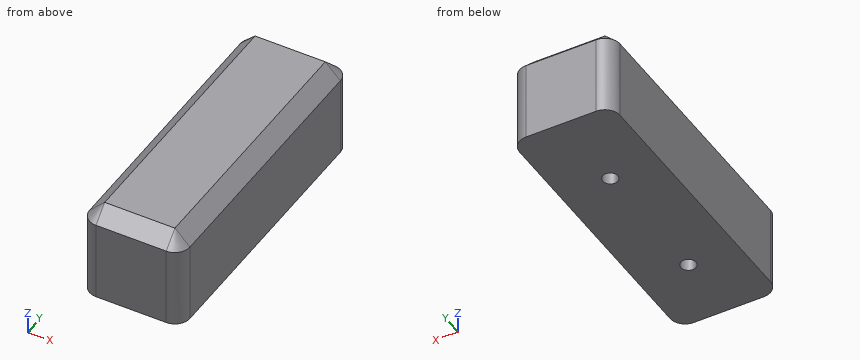
```python
from build123d import *

# Parameters (mm, degrees)
F0_W     = 20
F0_H     = 58
F1_DEPTH = 19
F2_R     = 1.5
F3_DEPTH = 17.000001
F4_R     = 3
F5_SIZE  = 3


with BuildPart() as f1:
    # F0 (on Top) → F1 (new body)
    with BuildSketch(Plane.XY):
        Rectangle(F0_W, F0_H)
    extrude(amount=F1_DEPTH)

    # F2 (on Top) → F3 (cut)
    with BuildSketch(Plane.XY):
        with Locations((0, 12)):
            Circle(F2_R)
        with Locations((0, -15)):
            Circle(F2_R)
    extrude(amount=F3_DEPTH, mode=Mode.SUBTRACT)

    # F4
    f4_edges = [f1.edges().sort_by_distance(p)[0] for p in [
        (-10, 29, 9.5),
        (10, 29, 9.5),
        (-10, -29, 9.5),
        (10, -29, 9.5),
    ]]
    fillet(f4_edges, radius=F4_R)

    # F5
    f5_edges = [f1.edges().sort_by_distance(p)[0] for p in [
        (-10, 0, 19),
    ]]
    chamfer(f5_edges, length=F5_SIZE)


solid = f1.part
```
Build history of the part. All positions in model axes, mm. Round coordinates to 2 decimals unless told otherwise and drop trailing zeros. Write each loop counter-clockwise with the first axis right and the second up, starting at its lowest first coordinate (ties: lowest second). Pieces come first, ordered by that corner, then holes.
1) Pin check, flat tip, straight feed: pin 1 (1.5 mm diameter, centred on x = 0.5, y = -15, fed in from -Z). Stop position of the tip, or through.
2) Band-saw the part on B-B, the plane x = 0. List the corners of the cut face in (y, z), and give its area (3 significant figures).
3) Band-saw the part on D-D, the plane y = 21. List the corners of the cut face in (x, z), and give its area (3 significant figures).
4) Drill centre lines: probe 1 along Y at (x, z) = (0, 11.5); probe 2 along X at (y, z) = (11, 14); probe 3 along Z at (x, y) = (0.5, 12). Where is each one in solid material? Low to high.
5) Band-saw the part on A-A, the plane z = 10. List the corners of the cut face in (x, y).
6) Band-saw the part on C-C, the plane y = -15. List the corners of the cut face in (x, z), and give its area (3 significant figures).
Ans:
1. pin 1: stops at z = 17
2. outline: (-29, 0) - (-16.5, 0) - (-16.5, 17) - (-13.5, 17) - (-13.5, 0) - (10.5, 0) - (10.5, 17) - (13.5, 17) - (13.5, 0) - (29, 0) - (29, 16) - (26, 19) - (-26, 19) - (-29, 16) - close
2. area: 991 mm2
3. outline: (-10, 0) - (10, 0) - (10, 16) - (7, 19) - (-7, 19) - (-10, 16) - close
3. area: 371 mm2
4. probe 1: y = -29 to -16.5, -13.5 to 10.5, 13.5 to 29
4. probe 2: x = -10 to -1.12, 1.12 to 10
4. probe 3: z = 17 to 19
5. outline: (-10, -26) arc R3 ccw to (-7, -29) - (7, -29) arc R3 ccw to (10, -26) - (10, 26) arc R3 ccw to (7, 29) - (-7, 29) arc R3 ccw to (-10, 26) - close; hole circle Ø3 at (0, -15); hole circle Ø3 at (0, 12)
6. outline: (-10, 0) - (-1.5, 0) - (-1.5, 17) - (1.5, 17) - (1.5, 0) - (10, 0) - (10, 16) - (7, 19) - (-7, 19) - (-10, 16) - close
6. area: 320 mm2
